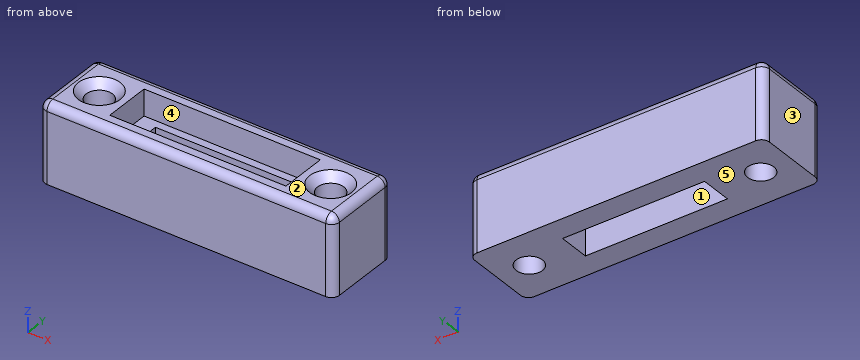
from build123d import *

# Parameters (mm, degrees)
F0_W           = 27
F0_H           = 6
F1_DEPTH       = 15
F3_R           = 1.5
F2_W           = 33.5
F2_H           = 9
F2_W_2         = 27
F2_H_2         = 6
F4_DEPTH       = 5
F5_D           = 5
F5_CSINK_D     = 8
F5_CSINK_ANGLE = 90


with BuildPart() as f1:
    # F0 (on Top) → F1 (new body)
    with BuildSketch(Plane.XY):
        with BuildLine():
            Line((-26.5, -7.5), (26.5, -7.5))
            ThreePointArc((26.5, -7.5), (27.5606601718, -7.0606601718), (28, -6))
            Line((28, -6), (28, 6))
            ThreePointArc((28, 6), (27.5606601718, 7.0606601718), (26.5, 7.5))
            Line((26.5, 7.5), (-26.5, 7.5))
            ThreePointArc((-26.5, 7.5), (-27.5606601718, 7.0606601718), (-28, 6))
            Line((-28, 6), (-28, -6))
            ThreePointArc((-28, -6), (-27.5606601718, -7.0606601718), (-26.5, -7.5))
        make_face()
        Rectangle(F0_W, F0_H, mode=Mode.SUBTRACT)
    extrude(amount=F1_DEPTH)

    # F3
    f3_edges = [f1.edges().sort_by_distance(p)[0] for p in [
        (0, -7.5, 15),
        (27.56066, -7.06066, 15),
        (28, 0, 15),
        (27.56066, 7.06066, 15),
        (0, 7.5, 15),
        (-27.56066, 7.06066, 15),
        (-28, 0, 15),
        (-27.56066, -7.06066, 15),
        (13.5, 0, 15),
        (0, -3, 15),
        (-13.5, 0, 15),
        (0, 3, 15),
    ]]
    fillet(f3_edges, radius=F3_R)

    # F2 (on face) → F4 (cut)
    with BuildSketch(Plane.XY.offset(15)):
        Rectangle(F2_W, F2_H)
        Rectangle(F2_W_2, F2_H_2, mode=Mode.SUBTRACT)
    extrude(amount=-F4_DEPTH, mode=Mode.SUBTRACT)

    # F5 (through all)
    with Locations(Plane.XY.offset(15)):
        with Locations((-22, 0), (22, 0)):
            CounterSinkHole(F5_D / 2, F5_CSINK_D / 2, counter_sink_angle=F5_CSINK_ANGLE)


solid = f1.part
Check sheet for the modelled part. Datum: model origin and axes. Units: mm. Face numbers are marked on the shaded views. A direction names the side the tool comes from. Give positions to 0.01 mm unless a question says otherwise; leave off trailing zeros. Loops run counter-clockwise (first coordinate to the right, second up) from the corner with the lowest first, then second, coordinate; pieces in that order, holes last. Notation, with made-up numbers: M -25,-4.5 L -16,-4.5 A19 cw -16,29.5 Z; hole C 52,16 d8. An arc over 180 degrees is marked long. Use a Markdown table: item, result. Add a question column.
Q1. Tool access check on the marked faces 4 and 5. Record the directions out of +Z, -Z, +X, -X, +Y, -Y that give a thin tool (end or side, any length) a straight path to the whole face; none if there is none.
Q2. Sectioned sample at C-C, the plane z = 4. Record the cut outline in (x, y).
Q3. Go/stop test with flat-tipped pins: pin 1 (6.5 mm diameter, centred on x = 22, y = 0, fed in from +Z); pin 2 (6 mm diameter, centred on x = -22, y = 0, fed in from +Z). Record where each tip stops, or that it passes through.
Q4. Sectioned sample at B-B, the plane y = 0. Record the cut outline in (x, z).
Q5. Mould release check, pull along X, two halves, no side actions. Record for the marked faces 1, 2 and 3: pulls with the +X half, pulls with the -X half, needs draft (parallel to the pull), parting line crosses it, or undercut.
Q6. Sectioned sample at A-A, the plane x = -22. Record the cut outline in (y, z).
Q7. Scan lines: line 1 along X through (y, z) = (-0.25, 4); line 2 along X through (y, z) = (-1.5, 6.25); line 3 along Y through (x, z) = (-22, 3.5). Record each from-to range of solid material in increasing order. Write a range as [from, to].
Q8. Sectioned sample at D-D, the plane x = 10. Record the cut outline in (y, z).
Verdict:
| question | item | result |
|---|---|---|
| 1 | face 4 | +Z |
| 1 | face 5 | -Z, +X, -X, +Y, -Y |
| 2 | outline | M -28,-6 A1.5 ccw -26.5,-7.5 L 26.5,-7.5 A1.5 ccw 28,-6 L 28,6 A1.5 ccw 26.5,7.5 L -26.5,7.5 A1.5 ccw -28,6 Z; hole C -22,0 d5; hole M -13.5,-3 L 13.5,-3 L 13.5,3 L -13.5,3 Z; hole C 22,0 d5 |
| 3 | pin 1 | z = 14.25 |
| 3 | pin 2 | z = 14 |
| 4 | outline | M -28,0 L -24.5,0 L -24.5,13.5 L -26,15 L -26.5,15 A1.5 ccw -28,13.5 Z; M -19.5,0 L -13.5,0 L -13.5,10 L -16.75,10 L -16.75,15 L -18,15 L -19.5,13.5 Z; M 13.5,0 L 19.5,0 L 19.5,13.5 L 18,15 L 16.75,15 L 16.75,10 L 13.5,10 Z; M 24.5,0 L 28,0 L 28,13.5 A1.5 ccw 26.5,15 L 26,15 L 24.5,13.5 Z |
| 5 | face 1 | undercut |
| 5 | face 2 | needs draft |
| 5 | face 3 | pulls with the -X half |
| 6 | outline | M -7.5,0 L -2.5,0 L -2.5,13.5 L -4,15 L -6,15 A1.5 ccw -7.5,13.5 Z; M 2.5,0 L 7.5,0 L 7.5,13.5 A1.5 ccw 6,15 L 4,15 L 2.5,13.5 Z |
| 7 | line 1 | [-28, -24.49], [-19.51, -13.5], [13.5, 19.51], [24.49, 28] |
| 7 | line 2 | [-28, -24], [-20, -13.5], [13.5, 20], [24, 28] |
| 7 | line 3 | [-7.5, -2.5], [2.5, 7.5] |
| 8 | outline | M -7.5,0 L -3,0 L -3,10 L -4.5,10 L -4.5,15 L -6,15 A1.5 ccw -7.5,13.5 Z; M 3,0 L 7.5,0 L 7.5,13.5 A1.5 ccw 6,15 L 4.5,15 L 4.5,10 L 3,10 Z |
